from build123d import *

# Parameters (mm, degrees)
F1_DEPTH = 6


with BuildPart() as f1:
    # F0 (on Front) → F1 (new body)
    with BuildSketch(Plane.XZ):
        with BuildLine():
            Line((-150, -115), (150, -115))
            Line((150, -115), (150, -32.871023))
            Line((150, -32.871023), (158, -32.871023))
            ThreePointArc((158, -32.871023), (165.071068, -29.942091), (168, -22.871023))
            Line((168, -22.871023), (168, 22.871023))
            ThreePointArc((168, 22.871023), (165.071068, 29.942091), (158, 32.871023))
            Line((158, 32.871023), (150, 32.871023))
            Line((150, 32.871023), (150, 115))
            Line((150, 115), (-150, 115))
            Line((-150, 115), (-150, -115))
        make_face()
    extrude(amount=F1_DEPTH)


solid = f1.part
Read the model definition and answer for the solid it produces. Units are mm, in the model's axes. A direction names the side the tool comes from. Give positions to 0.01 mm unless a question says otherwise; leave off trailing zeros. Write each loop counter-clockwise with the first axis right and the second up, starting at its lowest first coordinate (ties: lowest second). Pieces come first, ordered by that corner, then holes. Notation, with made-up numbers: M -38.75,50 L -6.75,50 A35 ccw -6.75,85 Z; hole C 88,70.5 d4. An arc over 180 degrees is marked long. One line per item, written item: value. Start each with the question number.
(1) A tool of negligible diameter and unlimited length cuts with its end or side. For faces 1 (the flat face through (150, -3, -75)), 2 (the flat face through (-150, -3, 2)), 3 (the flat face through (154, -3, 32.871)), from which of +Z, -Z, +X, -X, +Y, -Y can it reach the whole face along a straight path? Write none if from no direction.
(2) Find section B-B (z = -37.5). Determine the outline of the cut face in (x, y).
(3) Find the intervals of material crossed by line 1 (X direction, y = -4.1, z = 52.5); line 2 (X direction, y = -1.85, z = 28.5), in increasing order.
(4) Find section A-A (y = -1.1). Determine the outline of the cut face in (x, z).
(5) A flat-ended cylindrical pin translates along its axis: pin 1 Ø3 at (y, z) = (-1.5, -29) entering from +X. Find the tip coordinate at first contact, or state that the pin passes through.
Results below:
1. face 1: -Z, +X, +Y, -Y
1. face 2: +Z, -Z, -X, +Y, -Y
1. face 3: +Z, +X, +Y, -Y
2. outline: M -150,-6 L 150,-6 L 150,0 L -150,0 Z
3. line 1: x = -150 to 150
3. line 2: x = -150 to 166.27
4. outline: M -150,-115 L 150,-115 L 150,-32.87 L 158,-32.87 A10 ccw 168,-22.87 L 168,22.87 A10 ccw 158,32.87 L 150,32.87 L 150,115 L -150,115 Z
5. pin 1: stops at x = 166.86
